```python
from build123d import *

# Parameters (mm, degrees)
SCHIZZO1_W                   = 30
SCHIZZO1_H                   = 53
ESTRUSIONE_ESTRUSIONE1_DEPTH = 3
SCHIZZO3_W                   = 10
SCHIZZO3_H                   = 45
SCHIZZO3_W_2                 = 20
ESTRUSIONE_ESTRUSIONE2_DEPTH = 3
SCHIZZO5_R                   = 6
TAGLIO_ESTRUSIONE1_DEPTH     = 85.055041491


with BuildPart() as part:
    # Schizzo1 → Estrusione-Estrusione1 (new body)
    with BuildSketch(Plane.XY):
        with Locations((32.5, -23.5)):
            Rectangle(SCHIZZO1_W, SCHIZZO1_H)
    extrude(amount=ESTRUSIONE_ESTRUSIONE1_DEPTH)

    # Schizzo3 → Estrusione-Estrusione2 (add)
    with BuildSketch(Plane.XY.offset(3)):
        with Locations((12.5, -22.5)):
            Rectangle(SCHIZZO3_W, SCHIZZO3_H)
        with Locations((57.5, -22.5)):
            Rectangle(SCHIZZO3_W_2, SCHIZZO3_H)
    extrude(amount=-ESTRUSIONE_ESTRUSIONE2_DEPTH)

    # Schizzo5 → Taglio-Estrusione1 (cut, through all)
    with BuildSketch(Plane.XY.offset(3)):
        with Locations((27.15, -27.9)):
            Circle(SCHIZZO5_R)
    extrude(amount=-TAGLIO_ESTRUSIONE1_DEPTH, mode=Mode.SUBTRACT)


solid = part.part
```
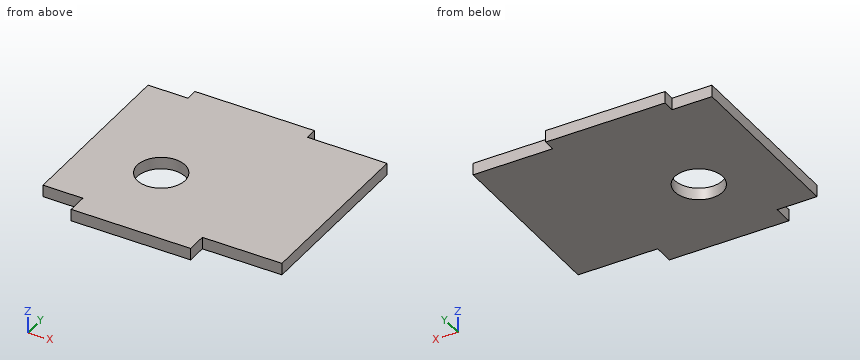
For this review, take the finished solid that the model builds, in its own axes (mm). Coordinates: 2 decimals unless noted, no trailing zeros. Loops run counter-clockwise (first coordinate to the right, second up) from the corner with the lowest first, then second, coordinate; pieces in that order, holes last.
1. For line 1 (Y direction, x = 27.15, z = 1.75); line 2 (Y direction, x = 55, z = 2.1); line 3 (X direction, y = 1, z = 2.45), list the stretches that pass through material, from the lowest coordinate up.
2. Insertion check: P1, Ø0.9, axis at y = -48, z = 1.5, coming from the -X side; P2, Ø1.5, axis at x = 14, z = 1, coming from the +Y side; P3, Ø1, axis at x = 60, y = -2.5, coming from the -Z side. Each pin has a flat end and moves straight along its axis. Give the tip position at first contact, or say it passes through.
3. Add section B-B, the plane y = -27.9. Give the boundary of the cut face in (x, z), then the cut area to 3 significant figures.
4. Add section D-D, the plane x = 50.5. Give the boundary of the cut face in (y, z).
5. Add section A-A, the plane x = 27.15. Give the boundary of the cut face in (y, z), then the cut area to 3 significant figures.
6. Add section C-C, the plane z = 0.95. Give the boundary of the cut face in (x, y).
Result:
1. line 1: y = -50 to -33.9, -21.9 to 3
1. line 2: y = -45 to 0
1. line 3: x = 17.5 to 47.5
2. P1: stops at x = 17.5
2. P2: stops at y = 0
2. P3: stops at z = 0
3. outline: (7.5, 0) - (21.15, 0) - (21.15, 3) - (7.5, 3) - close; (33.15, 0) - (67.5, 0) - (67.5, 3) - (33.15, 3) - close
3. area: 144 mm2
4. outline: (-45, 0) - (0, 0) - (0, 3) - (-45, 3) - close
5. outline: (-50, 0) - (-33.9, 0) - (-33.9, 3) - (-50, 3) - close; (-21.9, 0) - (3, 0) - (3, 3) - (-21.9, 3) - close
5. area: 123 mm2
6. outline: (7.5, -45) - (17.5, -45) - (17.5, -50) - (47.5, -50) - (47.5, -45) - (67.5, -45) - (67.5, 0) - (47.5, 0) - (47.5, 3) - (17.5, 3) - (17.5, 0) - (7.5, 0) - close; hole circle Ø12 at (27.15, -27.9)
